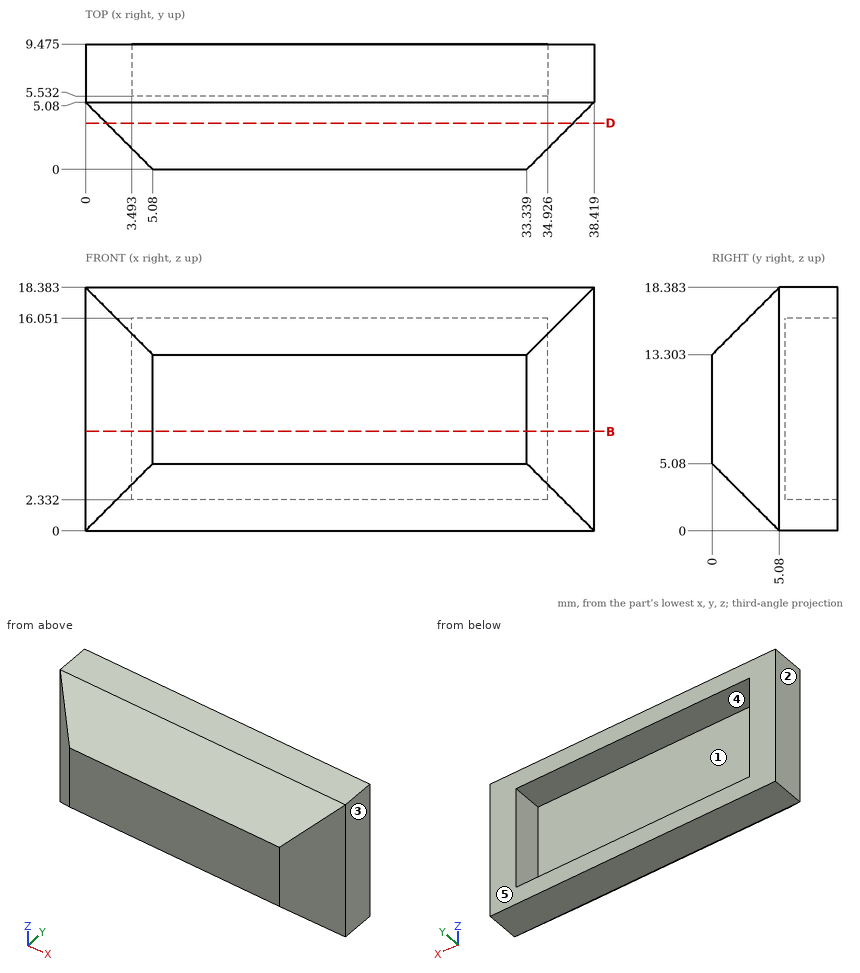
The figure shows three views and two pictorial views of one solid part (mm, origin at its lowest corner). Answer the questions. A direction names the side the tool comes from. Coordinates: 2 decimals unless noted, no trailing zeros. Loops run counter-clockwise (first coordinate to the right, second up) from the corner with the lowest first, then second, coordinate; pieces in that order, holes last.
(1) The part is cut by section B-B (z = 7.5). Determine the outline of the cut face in (x, y) (1 decimal).
Solution:
outline: (0, 5.1) - (5.1, 0) - (33.3, 0) - (38.4, 5.1) - (38.4, 9.5) - (34.9, 9.5) - (34.9, 5.5) - (3.5, 5.5) - (3.5, 9.5) - (0, 9.5) - close
(2) The part is cut by section D-D (y = 3.5). Determine the outline of the cut face in (x, z).
Solution:
outline: (1.58, 1.58) - (36.84, 1.58) - (36.84, 16.8) - (1.58, 16.8) - close
(3) Flat-ended cylindrical pins translate along their axes: pin 1 Ø7 at (x, z) = (19.5, 10.5) entering from +Y; pin 2 Ø4.5 at (x, y) = (16, 7.5) entering from -Z; pin 3 Ø3 at (x, z) = (33, 15.5) entering from -Y. Find the tip coordinate at first contact, or state that the pin passes through.
Solution:
pin 1: stops at y = 5.53
pin 2: stops at z = 0
pin 3: stops at y = 0.7
(4) A tool of negligible diameter and unlimited length cuts with its end or side. For the marked faces 4 and 5, from which of +Z, -Z, +X, -X, +Y, -Y can it reach the whole face along a straight path? Write none if from no direction.
Solution:
face 4: +Y
face 5: +Z, -Z, +X, -X, +Y
(5) The mould has two halves that part along X. Classify the marked faces 1, 2 and 3: released by +X, released by -X, zero draft, split by the parting line, or undercut.
Solution:
face 1: undercut
face 2: released by -X
face 3: released by +X
(6) Consider line 1 along X through (y, z) = (6.5, 14.75) (1 decimal); line 2 along Z through (x, y) = (18, 7); line 3 along Y through (x, z) = (23, 8.25). Determine where each line is inside the solid, lowest interval first.
Solution:
line 1: x = 0 to 3.5, 34.9 to 38.4
line 2: z = 0 to 2.33, 16.05 to 18.38
line 3: y = 0 to 5.53
